Input: part model. Units: mm. Frame: model coordinates. A direction names the side the tool comes from. Round coordinates to 2 decimals unless told otherwise and drop trailing zeros. Order: outer loops, then holes, each group sorted by start corner. A loop starts at its lowest first (then second) coordinate and runs counter-clockwise, first axis right, second up.
Item 1: Reachability of faces 1 (the flat face through (200, 10, 0)), 2 (the flat face through (365, 17.5, 4)), 3 (the flat face through (203, 10, 8)) from +Z, -Z, +X, -X, +Y, -Y: full face, straight path, thin tool, end or side. Return the list, or none.
Item 2: Cut plane A-A on z = 4.75. Give the number of separate pieces and of enclosed holes in the cut face, then the cut area to 3 significant figures.
Item 3: Line query: L1, parallel to Y at x = 39.85, z = 5.25; L2, parallel to Y at x = 39.85, z = 3.5; L3, parallel to X at y = 4.25, z = 5. Output: solid intervals per line, ascending.
Item 4: Cut plane B-B on x = 286.5. Output: boundary loops of the cut face in (y, z).
Item 5: First-contact query: pin 1 (2 mm diameter, centred on x = 282.5, y = 10.5, fed in from -Z); pin 2 (5 mm diameter, centred on y = 7, z = 7, fed in from +X); pin 3 (2.5 mm diameter, centred on x = 366, z = 4, fed in from +Y). Flat tips, straight axial feed; report the tip coordinate or a pass-through.
Item 6: Mould query, pull axis Y, two halves, no side actions, for faces 4 (the flat face through (200, 0, 5)), 5 (the flat face through (365, 10, 8)), 6 (the flat face through (365, 7.5, 4)). Classes: released by +Y, released by -Y, zero draft, split by the parting line, or undercut.
```python
from build123d import *

# Parameters (mm, degrees)
ESQUISSE1_R             = 2.5
ESQUISSE1_R_2           = 2
BOSS_EXTRU_1_DEPTH      = 10
CONG_1_R                = 10
TROU_TARAUD_M5X0_81_D   = 4.2
ESQUISSE5_W             = 10.1
ESQUISSE5_H             = 20
ESQUISSE5_W_2           = 20
ENL_V_MAT_EXTRU_1_DEPTH = 2
ESQUISSE6_R             = 3
ENL_V_MAT_EXTRU_3_DEPTH = 406.766586229


with BuildPart() as part:
    # Esquisse1 → Boss.-Extru.1 (new body)
    with BuildSketch(Plane.XY):
        Polygon((0, 20), (0, 0), (60, 0), (385.15, 0), (405.15, 0), (405.15, 20), (385.15, 20), (60, 20), align=None)
        with Locations((202.575, 15)):
            Circle(ESQUISSE1_R, mode=Mode.SUBTRACT)
        with Locations((202.575, 5)):
            Circle(ESQUISSE1_R, mode=Mode.SUBTRACT)
        with Locations((39.85, 5)):
            Circle(ESQUISSE1_R, mode=Mode.SUBTRACT)
        with Locations((39.85, 15)):
            Circle(ESQUISSE1_R, mode=Mode.SUBTRACT)
        with Locations((222.575, 10)):
            Circle(ESQUISSE1_R_2, mode=Mode.SUBTRACT)
        with Locations((262.575, 10)):
            Circle(ESQUISSE1_R_2, mode=Mode.SUBTRACT)
        with Locations((302.575, 10)):
            Circle(ESQUISSE1_R_2, mode=Mode.SUBTRACT)
        with Locations((342.575, 10)):
            Circle(ESQUISSE1_R_2, mode=Mode.SUBTRACT)
        with Locations((182.575, 10)):
            Circle(ESQUISSE1_R_2, mode=Mode.SUBTRACT)
        with Locations((142.575, 10)):
            Circle(ESQUISSE1_R_2, mode=Mode.SUBTRACT)
        with Locations((102.575, 10)):
            Circle(ESQUISSE1_R_2, mode=Mode.SUBTRACT)
        with Locations((62.575, 10)):
            Circle(ESQUISSE1_R_2, mode=Mode.SUBTRACT)
        with BuildLine():
            Line((360.3, 17.5), (370.3, 17.5))
            ThreePointArc((370.3, 17.5), (372.8, 15), (370.3, 12.5))
            Line((370.3, 12.5), (360.3, 12.5))
            ThreePointArc((360.3, 12.5), (357.8, 15), (360.3, 17.5))
        make_face(mode=Mode.SUBTRACT)
        with BuildLine():
            Line((360.3, 2.5), (370.3, 2.5))
            ThreePointArc((370.3, 2.5), (372.8, 5), (370.3, 7.5))
            Line((370.3, 7.5), (360.3, 7.5))
            ThreePointArc((360.3, 7.5), (357.8, 5), (360.3, 2.5))
        make_face(mode=Mode.SUBTRACT)
    extrude(amount=BOSS_EXTRU_1_DEPTH)

    # Congé1
    cong_1_edges = [part.edges().sort_by_distance(p)[0] for p in [
        (0, 0, 5),
        (0, 20, 5),
        (405.15, 0, 5),
        (405.15, 20, 5),
    ]]
    fillet(cong_1_edges, radius=CONG_1_R - 0.0001)  # a hair under: the kernel refuses the full size

    # Trou taraudé M5x0.81 (through all)
    with Locations(Plane.XY.offset(10)):
        with Locations((385.15, 10), (395.15, 10), (10, 10), (20, 10)):
            Hole(TROU_TARAUD_M5X0_81_D / 2)

    # Esquisse5 → Enlèv. mat.-Extru.1 (cut)
    with BuildSketch(Plane.XY.offset(10)):
        with Locations((202.575, 10)):
            Rectangle(ESQUISSE5_W, ESQUISSE5_H)
        with Locations((365.3, 10)):
            Rectangle(ESQUISSE5_W_2, ESQUISSE5_H)
        with Locations((39.85, 10)):
            Rectangle(ESQUISSE5_W, ESQUISSE5_H)
    extrude(amount=-ENL_V_MAT_EXTRU_1_DEPTH, mode=Mode.SUBTRACT)

    # Esquisse6 → Enlèv. mat.-Extru.3 (cut, through all)
    with BuildSketch(Plane(origin=(0, 0, 0), x_dir=(0, 0, -1), z_dir=(1, 0, 0))):
        with Locations((-5, 21)):
            Circle(ESQUISSE6_R)
    extrude(amount=ENL_V_MAT_EXTRU_3_DEPTH, mode=Mode.SUBTRACT)


solid = part.part
```
From the geometry:
1. face 1: -Z, +X, -X, +Y, -Y
1. face 2: +Z, -Z
1. face 3: +Z, +Y, -Y
2. separate pieces: 1
2. enclosed holes: 18
2. area: 6,860 mm2
3. L1: y = 0 to 2.5, 7.5 to 12.5, 17.5 to 18.01
3. L2: y = 0 to 2.5, 7.5 to 12.5, 17.5 to 18.4
3. L3: x = 1.82 to 37.47, 42.23 to 200.19, 204.96 to 357.92, 372.68 to 403.33
4. outline: (0, 0) - (20, 0) - (20, 2.17) arc R3 cw to (20, 7.83) - (20, 10) - (0, 10) - close
5. pin 1: stops at z = 0
5. pin 2: stops at x = 405.14
5. pin 3: stops at y = 19.02
6. face 4: released by -Y
6. face 5: zero draft
6. face 6: undercut
